Could you check a few things on this model? Use its own coordinates, in mm. A direction names the side the tool comes from. Give positions to 0.01 mm unless a question says otherwise; leave off trailing zeros. Write each loop counter-clockwise with the first axis right and the second up, starting at its lowest first coordinate (ties: lowest second). Pieces come first, ordered by that corner, then holes. Notation, with made-up numbers: M 41.25,-26 L 77.25,-26 A24 ccw 77.25,9 Z; hole C -9,29.5 d3. An arc over 180 degrees is marked long. Use one line per item in the form item = value.
from build123d import *

# Parameters (mm, degrees)
F0_W           = 30
F0_H           = 15
F1_DEPTH       = 5
F2_W           = 30
F2_H           = 5
F3_DEPTH       = 50
F4_DEPTH       = 10
F5_DEPTH       = 10
F6_DEPTH       = 4
F8_D           = 5.1054
F8_DEPTH       = 10
F8_CSINK_D     = 10.4394
F8_CSINK_ANGLE = 82
F8_TIP         = 1.5338169022
F9_W           = 40
F9_H           = 5
F10_DEPTH      = 19.001


with BuildPart() as f1:
    # F0 (on Top) → F1 (new body)
    with BuildSketch(Plane.XY):
        Rectangle(F0_W, F0_H)
    extrude(amount=F1_DEPTH)

    # F2 (on face) → F3 (join)
    with BuildSketch(Plane.XY.offset(5)):
        with Locations((0, 5)):
            Rectangle(F2_W, F2_H)
    extrude(amount=F3_DEPTH)

    # F4 (add): a face of the model
    f4_faces = [f1.faces().sort_by_distance(p)[0] for p in [
        (-15, 3.8461538462, 23.6538461538),
    ]]
    extrude(f4_faces, amount=F4_DEPTH)

    # F5 (add): a face of the model
    f5_faces = [f1.faces().sort_by_distance(p)[0] for p in [
        (15, 3.8461538462, 23.6538461538),
    ]]
    extrude(f5_faces, amount=F5_DEPTH)

    # F6 (add): a face of the model
    f6_faces = [f1.faces().sort_by_distance(p)[0] for p in [
        (0, -7.5, 2.5),
    ]]
    extrude(f6_faces, amount=F6_DEPTH)

    # F8
    with Locations(Plane.XY.offset(5)):
        with Locations((15, -4.5), (-15, -4.5)):
            CounterSinkHole(F8_D / 2, F8_CSINK_D / 2, depth=F8_DEPTH, counter_sink_angle=F8_CSINK_ANGLE)
            with Locations((0, 0, -(F8_DEPTH + F8_TIP / 2))):  # 118° drill point
                Cone(0, F8_D / 2, F8_TIP, mode=Mode.SUBTRACT)

    # F9 (on face) → F10 (cut, through all)
    with BuildSketch(Plane(origin=(0, 7.5, 0), x_dir=(-1, 0, 0), z_dir=(0, 1, 0))):
        with Locations((0, 27.5)):
            Rectangle(F9_W, F9_H)
    extrude(amount=-F10_DEPTH, mode=Mode.SUBTRACT)


solid = f1.part
1) If I drill on L1, parallel to X at y = -4.5, z = 0.75; L2, parallel to Y at x = 15, z = 1.1; L3, parallel to X at y = 4.25, z = 28, over which ranges is the centre line in solid material (lowest first)?
Checked values:
L1 = -25 to -17.55, -12.45 to 12.45, 17.55 to 25
L2 = -11.5 to -7.05, -1.95 to 7.5
L3 = -25 to -20, 20 to 25
2) I want a section at B-B, the plane y = 4. Please give me the cut outline in (x, z), plus the area to 3 significant figures.
Checked values:
outline = M -25,0 L 25,0 L 25,55 L -25,55 Z; hole M -20,25 L 20,25 L 20,30 L -20,30 Z
area = 2,550 mm2
3) I want a section at D-D, the plane x = 15. Please give me the cut outline in (y, z).
Checked values:
outline = M -11.5,0 L -7.05,0 L -7.05,1.93 L -9.72,5 L -11.5,5 Z; M -1.95,0 L 7.5,0 L 7.5,25 L 2.5,25 L 2.5,5 L 0.72,5 L -1.95,1.93 Z; M 2.5,30 L 7.5,30 L 7.5,55 L 2.5,55 Z
4) Thinking about a two-plate mould opening in Y: for faces 1 (the flat face through (0, 7.5, 34)), 2 (the flat face through (20, 5, 27)), 3 (the conical face through (-16.24, -6.88, 2.08)), 4 (the cylindrical face through (12.565, -3.733, 0.952)), which applies, released by +Y, released by -Y, zero draft, split by the parting line, or undercut?
Checked values:
face_1 = released by +Y
face_2 = zero draft
face_3 = undercut
face_4 = undercut
5) For pin 1 Ø10 at (y, z) = (-4.5, 33.5) entering from +X; pin 2 Ø7 at (x, y) = (9, -2.5) entering from +Z; pin 3 Ø1.5 at (x, z) = (4, 13.5) entering from -Y, each with a flat end and sliding along its axis, tell me the tip position at first contact or that it passes through.
Checked values:
pin_1 = through
pin_2 = 5
pin_3 = 2.5
6) I want a section at A-A, the plane x = -2.5. Please give me the cut outline in (y, z), plus the area to 3 significant figures.
Checked values:
outline = M -11.5,0 L 7.5,0 L 7.5,25 L 2.5,25 L 2.5,5 L -11.5,5 Z; M 2.5,30 L 7.5,30 L 7.5,55 L 2.5,55 Z
area = 320 mm2
7) I want a section at C-C, the plane z = 28. Please give me the cut outline in (x, y), plus the area to 3 significant figures.
Checked values:
outline = M -25,2.5 L -20,2.5 L -20,7.5 L -25,7.5 Z; M 20,2.5 L 25,2.5 L 25,7.5 L 20,7.5 Z
area = 50.0 mm2
8) For faces 5 (the flat face through (0, 5, 25)), 6 (the flat face through (0, -4, 5)), 7 (the flat face through (25, 3, 21)), which set-ups out of +Z, -Z, +X, -X, +Y, -Y let a thin tool reach every point of the face, with its end or its side?
Checked values:
face_5 = +Y, -Y
face_6 = +Z, +X, -X, -Y
face_7 = +Z, -Z, +X, +Y, -Y
